```python
from build123d import *

# Parameters (mm, degrees)
F0_W     = 20
F0_H     = 19.999998
F1_DEPTH = 20
F2_R     = 7.5
F3_DEPTH = 20.001
F4_W     = 20
F4_H     = 20
F5_DEPTH = 32.5


with BuildPart() as f1:
    # F0 (on Right) → F1 (new body)
    with BuildSketch(Plane.YZ):
        Rectangle(F0_W, F0_H)
    extrude(amount=F1_DEPTH)

    # F2 (on face) → F3 (cut, through all)
    with BuildSketch(Plane.YZ.offset(20)):
        Circle(F2_R)
    extrude(amount=-F3_DEPTH, mode=Mode.SUBTRACT)

    # F4 (on face) → F5 (join)
    with BuildSketch(Plane.XY.offset(9.999999)):
        with Locations((10, 0)):
            Rectangle(F4_W, F4_H)
    extrude(amount=F5_DEPTH)


solid = f1.part
```
Work out the finished part from the listing and answer in its coordinate system (mm). Round coordinates to 2 decimals unless told otherwise and drop trailing zeros. Loops run counter-clockwise (first coordinate to the right, second up) from the corner with the lowest first, then second, coordinate; pieces in that order, holes last. Notation, with made-up numbers: (24, -24.75) -> (71, -24.75) arc R18 cw to (71, 0.25) -> close; hole circle Ø11 at (27.5, 40). An arc over 180 degrees is marked (long way). Write each question's results on one line, items separated by ' | '. Start each with the question number.
1. Section A-A (z = 0) is taken. Determine the outline of the cut face in (x, y), plus the area to 3 significant figures.
2. Find the intervals of material crossed by probe 1 along Z at (x, y) = (5.25, 0); probe 2 along Z at (x, y) = (15.75, 3); probe 3 along Y at (x, z) = (7.25, 2), in increasing order. Write a range as from..to.
3. Section B-B (y = 0) is taken. Determine the outline of the cut face in (x, z).
4. Section C-C (x = 11.25) is taken. Determine the outline of the cut face in (y, z), plus the area to 3 significant figures.
5. For a pull along Y with two mould halves and no side action, classify faces 1 (the face through (10, 10, 16)), 2 (the face through (10, -10, 16)), 3 (the face through (10.14, -7.493, 0.33)) as +Y half, -Y half, draft (parallel to the pull), parting line (faces both ways), or undercut.
6. Given pin 1 Ø8 at (y, z) = (4.5, 1) entering from -X, flat-ended and moving along its own axis, determine where the tip first touches the part or whether it passes through.
Evaluation:
1) outline: (0, -10) -> (20, -10) -> (20, -7.5) -> (0, -7.5) -> close; (0, 7.5) -> (20, 7.5) -> (20, 10) -> (0, 10) -> close | area: 100 mm2
2) probe 1: z = -10..-7.5, 7.5..42.5 | probe 2: z = -10..-6.87, 6.87..42.5 | probe 3: y = -10..-7.23, 7.23..10
3) outline: (0, -10) -> (20, -10) -> (20, -7.5) -> (0, -7.5) -> close; (0, 7.5) -> (20, 7.5) -> (20, 42.5) -> (0, 42.5) -> close
4) outline: (-10, -10) -> (10, -10) -> (10, 42.5) -> (-10, 42.5) -> close; hole circle Ø15 at (0, 0) | area: 873 mm2
5) face 1: +Y half | face 2: -Y half | face 3: undercut
6) pin 1: stops at x = 0
